Build history of the part. All positions in model axes, mm. A direction names the side the tool comes from. Give positions to 0.01 mm unless a question says otherwise; leave off trailing zeros. Write each loop counter-clockwise with the first axis right and the second up, starting at its lowest first coordinate (ties: lowest second). Pieces come first, ordered by that corner, then holes. Notation, with made-up numbers: (43, 25) -> (75, 25) arc R22 ccw to (75, 57) -> close; hole circle Ø6 at (81, 27). An arc over 180 degrees is marked (long way). Put each result on its own line as item: value. Start each with the question number.
Item 1: Flat gauge pins, fed straight in: pin 1 Ø23.5 at (x, y) = (-4.5, 34) entering from +Z; pin 2 Ø10 at (x, z) = (-8.5, -4) entering from +Y; pin 3 Ø6 at (x, z) = (13.5, -18) entering from -Y. Where does each tip first touch, or does it go through?
Item 2: Tool access for faces 4 (the flat face through (0, -10, 12.75)), 5 (the flat face through (9.75, -10, 0)), 6 (the flat face through (23.5, 17, -10)), 7 (the flat face through (-13.7, 43, -26)), 8 (the flat face through (0, 53, -26)): list every direction of +Z, -Z, +X, -X, +Y, -Y with a clear straight run to the whole face (end or side of a thin tool).
Item 3: Slice it at D-D, the plane x = -21. List the corners of the cut face in (y, z), plus the area to 3 significant figures.
Item 4: Slice it at A-A, the plane x = 0. List the corners of the cut face in (y, z), plus the area to 3 significant figures.
Item 5: Two-plate mould, pull along Y, no slides. Class faces 1 (the flat face through (0, 1, 27.5)), 2 (the flat face through (17.3, 43, -26)), 3 (the flat face through (-25.528, 27.65, 1.864)): pulls with the +Y half, pulls with the -Y half, needs draft (parallel to the pull), parting line crosses it, or undercut.
Item 6: Slice it at B-B, the plane y = 17.5. List the corners of the cut face in (x, z), plus the area to 3 significant figures.
Item 7: Drill centre lines: line 1 along X through (y, z) = (20, 9.5); line 2 along Z through (x, y) = (-11, -10); line 3 along Y through (x, z) = (10, 8.5). Where is each one in solid material? Low to high.
Item 8: Slice it at C-C, the plane z = -5. List the corners of the cut face in (x, y).
```python
from build123d import *

# Parameters (mm, degrees)
SKETCH1_W           = 25.5
SKETCH1_H           = 25.5
SKETCH1_W_2         = 19.5
SKETCH1_H_2         = 19.5
BOSS_EXTRUDE1_DEPTH = 20
SKETCH2_W           = 55
SKETCH2_H           = 55
BOSS_EXTRUDE2_DEPTH = 3
SKETCH3_W           = 55
SKETCH3_H           = 3
BOSS_EXTRUDE3_DEPTH = 50
BOSS_EXTRUDE4_DEPTH = 4
CUT_EXTRUDE1_DEPTH  = 80.178595592


with BuildPart() as part:
    # Sketch1 → Boss-Extrude1 (new body)
    with BuildSketch(Plane(origin=(0, 0, 0), x_dir=(1, 0, 0), z_dir=(0, 1, 0))):
        Rectangle(SKETCH1_W, SKETCH1_H)
        Rectangle(SKETCH1_W_2, SKETCH1_H_2, mode=Mode.SUBTRACT)
    extrude(amount=-BOSS_EXTRUDE1_DEPTH)

    # Sketch2 → Boss-Extrude2 (add)
    with BuildSketch(Plane(origin=(0, 0, 0), x_dir=(1, 0, 0), z_dir=(0, 1, 0))):
        Rectangle(SKETCH2_W, SKETCH2_H)
    extrude(amount=BOSS_EXTRUDE2_DEPTH)

    # Sketch3 → Boss-Extrude3 (add)
    with BuildSketch(Plane(origin=(0, 3, 0), x_dir=(1, 0, 0), z_dir=(0, 1, 0))):
        with Locations((0, 26)):
            Rectangle(SKETCH3_W, SKETCH3_H)
    extrude(amount=BOSS_EXTRUDE3_DEPTH)

    # Sketch4 → Boss-Extrude4 (add)
    with BuildSketch(Plane.ZY.offset(27.5)):
        Polygon((-24.5, 3), (27.5, 3), (-24.5, 53), align=None)
    boss_extrude4 = extrude(amount=-BOSS_EXTRUDE4_DEPTH)

    # Mirror1: Boss-Extrude4 across plane
    add(boss_extrude4.mirror(Plane(origin=(0, 0, 0), x_dir=(0, 0, 1), z_dir=(1, 0, 0))))

    # Sketch5 → Cut-Extrude1 (cut, through all)
    with BuildSketch(Plane.XY.offset(-24.5)):
        with BuildLine():
            Line((-17.3, 9.5), (-17.3, 14.5))
            ThreePointArc((-17.3, 14.5), (-15.5, 16.3), (-13.7, 14.5))
            Line((-13.7, 14.5), (-13.7, 9.5))
            ThreePointArc((-13.7, 9.5), (-15.5, 7.7), (-17.3, 9.5))
        make_face()
        with BuildLine():
            Line((13.7, 9.5), (13.7, 14.5))
            ThreePointArc((13.7, 14.5), (15.5, 16.3), (17.3, 14.5))
            Line((17.3, 14.5), (17.3, 9.5))
            ThreePointArc((17.3, 9.5), (15.5, 7.7), (13.7, 9.5))
        make_face()
        with BuildLine():
            Line((13.7, 40.5), (13.7, 45.5))
            ThreePointArc((13.7, 45.5), (15.5, 47.3), (17.3, 45.5))
            Line((17.3, 45.5), (17.3, 40.5))
            ThreePointArc((17.3, 40.5), (15.5, 38.7), (13.7, 40.5))
        make_face()
        with BuildLine():
            Line((-17.3, 40.5), (-17.3, 45.5))
            ThreePointArc((-17.3, 45.5), (-15.5, 47.3), (-13.7, 45.5))
            Line((-13.7, 45.5), (-13.7, 40.5))
            ThreePointArc((-13.7, 40.5), (-15.5, 38.7), (-17.3, 40.5))
        make_face()
        with BuildLine():
            Line((-12, 25), (-12, 30))
            ThreePointArc((-12, 30), (0, 42), (12, 30))
            Line((12, 30), (12, 25))
            ThreePointArc((12, 25), (0, 13), (-12, 25))
        make_face()
    extrude(amount=-CUT_EXTRUDE1_DEPTH, mode=Mode.SUBTRACT)


solid = part.part
```
Values follow:
1. pin 1: z = -24.5
1. pin 2: y = 3
1. pin 3: y = 0
2. face 4: +Z, +X, -X, -Y
2. face 5: -Y
2. face 6: +Z, +Y
2. face 7: +Z, -Z
2. face 8: +Z, -Z, +X, -X, +Y
3. outline: (0, -27.5) -> (53, -27.5) -> (53, -24.5) -> (3, -24.5) -> (3, 27.5) -> (0, 27.5) -> close
3. area: 315 mm2
4. outline: (-20, -12.75) -> (0, -12.75) -> (0, -27.5) -> (13, -27.5) -> (13, -24.5) -> (3, -24.5) -> (3, 27.5) -> (0, 27.5) -> (0, 12.75) -> (-20, 12.75) -> (-20, 9.75) -> (0, 9.75) -> (0, -9.75) -> (-20, -9.75) -> close; (42, -27.5) -> (53, -27.5) -> (53, -24.5) -> (42, -24.5) -> close
4. area: 348 mm2
5. face 1: needs draft
5. face 2: undercut
5. face 3: pulls with the +Y half
6. outline: (-27.5, -27.5) -> (-9.37, -27.5) -> (-9.37, -24.5) -> (-23.5, -24.5) -> (-23.5, 12.42) -> (-27.5, 12.42) -> close; (9.37, -27.5) -> (27.5, -27.5) -> (27.5, 12.42) -> (23.5, 12.42) -> (23.5, -24.5) -> (9.37, -24.5) -> close
6. area: 404 mm2
7. line 1: -27.5 to -23.5, 23.5 to 27.5
7. line 2: -12.75 to 12.75
7. line 3: -20 to 3
8. outline: (-27.5, 0) -> (-12.75, 0) -> (-12.75, -20) -> (-9.75, -20) -> (-9.75, 0) -> (9.75, 0) -> (9.75, -20) -> (12.75, -20) -> (12.75, 0) -> (27.5, 0) -> (27.5, 34.25) -> (23.5, 34.25) -> (23.5, 3) -> (-23.5, 3) -> (-23.5, 34.25) -> (-27.5, 34.25) -> close
